Drawing for the job (mm, zero at the part's lowest x, y, z). A direction names the side the tool comes from. Give positions to 0.01 mm unless a question says otherwise; leave off trailing zeros. Write each loop counter-clockwise with the first axis right and the second up, starting at its lowest first coordinate (ties: lowest second). Pieces come first, ordered by that corner, then holes. Notation, with made-up numbers: (-26, -24.75) - (27, -24.75) arc R16 ccw to (27, -17.75) - close; hole circle Ø8 at (19, -4). An arc over 180 degrees is marked (long way). Answer as a JSON object with one key per item and string values. Group by question number.
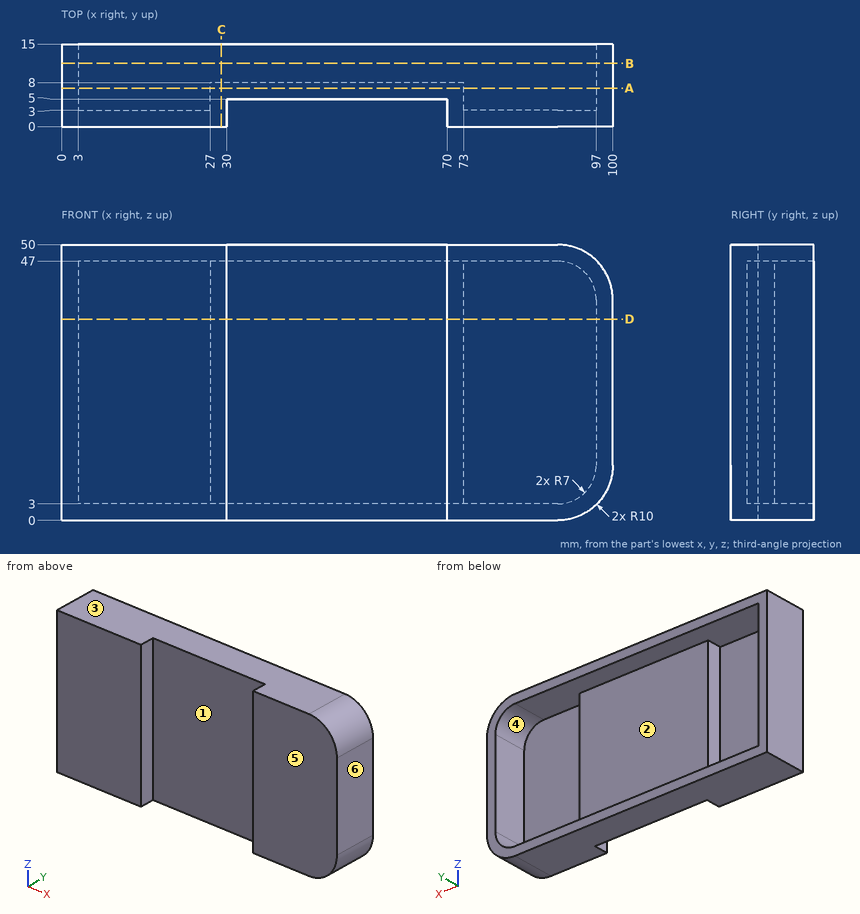
1) Drop flat-ended pins along their axis: P1, Ø2, axis at y = 3, z = 42.5, coming from the +X side; P2, Ø20, axis at x = 55.5, z = 32, coming from the -Y side; P3, Ø12, axis at x = 79.5, z = 26.5, coming from the +Y side. Give the stop position or say it passes through.
2) Mould opens along X. For the marked faces 4, 5 and 6 say: pulls with the +X half, pulls with the -X half, needs draft (parallel to the pull), parting line crosses it, or undercut.
3) Band-saw the part on B-B (y = 11.5). List the corners of the cut face in (x, z).
4) Which spindle directions (+Z, -Z, +X, -X, +Y, -Y) get a long thin tool onto all of the face, cutting with end or side? Do the marked faces 1, 2 and 3. Say none if no direction does.
5) Probe line 1 (X direction, y = 7, z = 40); line 2 (Z direction, x = 35, y = 13); line 3 (X direction, y = 8.75, z = 34). List the from-to ranges inside material, lowest first.
6) Band-saw the part on A-A (y = 7). List the corners of the cut face in (x, z), plus the area to 3 significant figures.
7) Band-saw the part on D-D (z = 36.5). List the corners of the cut face in (x, y), plus the area to 3 significant figures.
8) Band-saw the part on C-C (x = 29). List the corners of the cut face in (y, z), plus the area to 3 significant figures.
Verdict:
{
 "1": {"P1": "x = 99.89", "P2": "y = 5", "P3": "y = 3"},
 "2": {"face 4": "undercut", "face 5": "needs draft", "face 6": "pulls with the +X half"},
 "3": {"outline": "(0, 0) - (90, 0) arc R10 ccw to (100, 10) - (100, 40) arc R10 ccw to (90, 50) - (0, 50) - close; hole (3, 3) - (90, 3) arc R7 ccw to (97, 10) - (97, 40) arc R7 ccw to (90, 47) - (3, 47) - close"},
 "4": {"face 1": "+Z, -Z, -Y", "face 2": "+Y", "face 3": "+Z, +X, -X, +Y, -Y"},
 "5": {"line 1": "0 to 3, 27 to 73, 97 to 100", "line 2": "0 to 3, 47 to 50", "line 3": "0 to 3, 97 to 100"},
 "6": {"outline": "(0, 0) - (90, 0) arc R10 ccw to (100, 10) - (100, 40) arc R10 ccw to (90, 50) - (0, 50) - close; hole (3, 3) - (27, 3) - (27, 47) - (3, 47) - close; hole (73, 3) - (90, 3) arc R7 ccw to (97, 10) - (97, 40) arc R7 ccw to (90, 47) - (73, 47) - close", "area": "2,870 mm2"},
 "7": {"outline": "(0, 0) - (30, 0) - (30, 5) - (70, 5) - (70, 0) - (100, 0) - (100, 15) - (97, 15) - (97, 3) - (73, 3) - (73, 8) - (27, 8) - (27, 3) - (3, 3) - (3, 15) - (0, 15) - close", "area": "402 mm2"},
 "8": {"outline": "(0, 0) - (15, 0) - (15, 3) - (8, 3) - (8, 47) - (15, 47) - (15, 50) - (0, 50) - close", "area": "442 mm2"}
}
